Could you check a few things on this model? Use its own coordinates, in mm. A direction names the side the tool comes from. Give positions to 0.01 mm unless a question says otherwise; leave off trailing zeros. Write each loop counter-clockwise with the first axis right and the second up, starting at its lowest first coordinate (ties: lowest second). Pieces come first, ordered by that corner, then holes. Notation, with made-up numbers: M -39,-38.75 L -11,-38.75 A33 ccw -11,-7.75 Z; hole C 69,23 d6. An arc over 180 degrees is marked long. One line per item, written item: value.
```python
from build123d import *

# Parameters (mm, degrees)
BOSS_EXTRUDE1_DEPTH = 3.175


with BuildPart() as part:
    # Sketch1 → Boss-Extrude1 (new body)
    # profile 1 of 2: a face of its own
    with BuildSketch(Plane(origin=(0, 0, 0), x_dir=(1, 0, 0), z_dir=(0, 1, 0))):
        with BuildLine():
            Line((0, 0), (10.675, 0))
            Line((10.675, 0), (21.35, 0))
            Line((21.35, 0), (21.35, 20))
            Line((21.35, 20), (21.35, 23.75))
            ThreePointArc((21.35, 23.75), (20.1, 25), (21.35, 26.25))
            Line((21.35, 26.25), (21.35, 30))
            Line((21.35, 30), (0, 30))
            Line((0, 30), (0, 0))
        make_face()
        with BuildLine():
            ThreePointArc((12.175, 10), (11.735660172, 8.939339828), (10.675, 8.5))
            ThreePointArc((10.675, 8.5), (9.175, 10), (10.675, 11.5))
            ThreePointArc((10.675, 11.5), (11.735660172, 11.060660172), (12.175, 10))
        make_face(mode=Mode.SUBTRACT)
        with BuildLine():
            ThreePointArc((12.175, 20), (11.735660172, 18.939339828), (10.675, 18.5))
            ThreePointArc((10.675, 18.5), (9.614339828, 21.060660172), (12.175, 20))
        make_face(mode=Mode.SUBTRACT)
    # profile 2 of 2: a face of its own
    with BuildSketch(Plane(origin=(0, 0, 0), x_dir=(1, 0, 0), z_dir=(0, 1, 0))):
        with BuildLine():
            Line((21.35, 23.75), (21.35, 20))
            Line((21.35, 20), (26.35, 20))
            Line((26.35, 20), (26.35, 30))
            Line((26.35, 30), (21.35, 30))
            Line((21.35, 30), (21.35, 26.25))
            ThreePointArc((21.35, 26.25), (22.233883476, 25.883883476), (22.6, 25))
            ThreePointArc((22.6, 25), (22.233883476, 24.116116524), (21.35, 23.75))
        make_face()
    extrude(amount=BOSS_EXTRUDE1_DEPTH)


solid = part.part
```
1) If we section it at B-B, the plane z = -24.5: Write out the boundary of the cut face in (x, y) (3 decimals).
Outcome:
outline: M 0,0 L 20.204,0 L 20.204,3.175 L 0,3.175 Z; M 22.496,0 L 26.35,0 L 26.35,3.175 L 22.496,3.175 Z
2) On a 3-axis mill with a long thin cutter (end or side, diameter ignored), from which of +Z, -Z, +X, -X, +Y, -Y can I reach the whole of each face in a straight line? I mean faces 1 (the face through (24, 2, -20)), 2 (the face through (10, 3.175, -15)). Say none if no direction works.
Outcome:
face 1: +Z, +X, +Y, -Y
face 2: +Z, -Z, +X, -X, +Y
3) I'm going to push flat-ended pins straight in: pin 1 (10 mm diameter, centred on x = 15, z = -7.5, fed in from -Y); pin 2 (1.6 mm diameter, centred on y = 1.5, z = -7, fed in from +X); pin 3 (1 mm diameter, centred on x = 22.5, y = 1.5, fed in from +Z). Where does each tip first touch, or does it pass through?
Outcome:
pin 1: stops at y = 0
pin 2: stops at x = 21.35
pin 3: stops at z = -20
4) If we section it at C-C, the plane y = 2.35: Write out the boundary of the cut face in (x, z) (3 decimals), then the cut area to 3 significant figures.
Outcome:
outline: M 0,-30 L 26.35,-30 L 26.35,-20 L 21.35,-20 L 21.35,0 L 0,0 Z; hole C 10.675,-20 d3; hole C 10.675,-10 d3; hole C 21.35,-25 d2.5
area: 671 mm^2
5) Please list where these lines run through material, in increasing order: L1, parallel to Z at x = 11, y = 1.15; L2, parallel to X at y = 0.9, z = -4.75; L3, parallel to Z at x = 24.25, y = 0.1. Write a range as from..to.
Outcome:
L1: z = -30..-21.46, -18.54..-11.46, -8.54..0
L2: x = 0..21.35
L3: z = -30..-20
6) If we section it at D-D, the plane x = 22: Write out the boundary of the cut face in (y, z) (3 decimals), then the cut area to 3 significant figures.
Outcome:
outline: M 0,-30 L 3.175,-30 L 3.175,-26.068 L 0,-26.068 Z; M 0,-23.932 L 3.175,-23.932 L 3.175,-20 L 0,-20 Z
area: 25.0 mm^2
7) If we section it at A-A, the plane x = 10: Write out the boundary of the cut face in (y, z) (3 decimals), then the cut area to 3 significant figures.
Outcome:
outline: M 0,-30 L 3.175,-30 L 3.175,-21.34 L 0,-21.34 Z; M 0,-18.66 L 3.175,-18.66 L 3.175,-11.34 L 0,-11.34 Z; M 0,-8.66 L 3.175,-8.66 L 3.175,0 L 0,0 Z
area: 78.2 mm^2
